Can you work these out from the drawing? Everything is in mm from the part's minimum corner. Round coordinates to 2 decimals unless told otherwise and drop trailing zeros. Loops run counter-clockwise (first coordinate to the right, second up) from the corner with the lowest first, then second, coordinate; pieces in that order, holes last. Notation, with made-up numbers: (28, 83.25) -> (51, 83.25) arc R16 ccw to (51, 92.25) -> close; hole circle Ø3 at (-18, 4.25). An arc over 180 degrees is marked (long way). One line per item, written item: value.
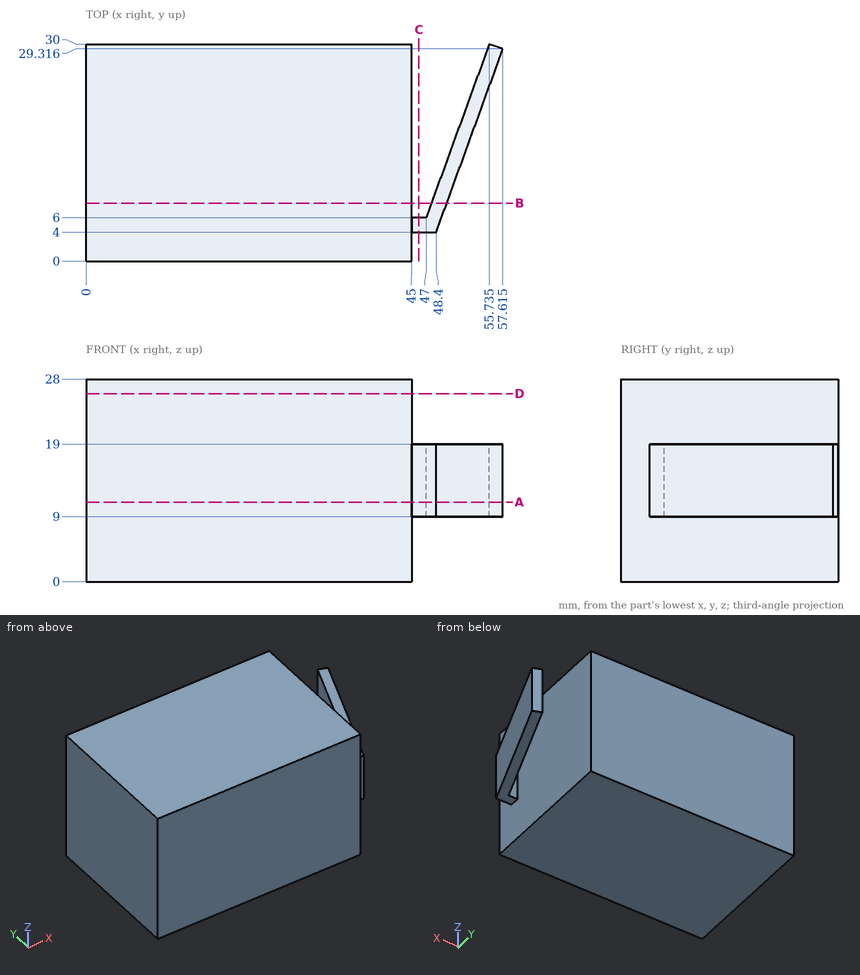
(1) If we section it at B-B, the plane y = 8: Please give me the cut outline in (x, z).
Recorded:
outline: (0, 0) -> (45, 0) -> (45, 28) -> (0, 28) -> close; (47.73, 9) -> (49.86, 9) -> (49.86, 19) -> (47.73, 19) -> close
(2) If we section it at D-D, the plane z = 26: Please give me the cut outline in (x, y), then the cut area to 3 significant figures.
Recorded:
outline: (0, 0) -> (45, 0) -> (45, 30) -> (0, 30) -> close
area: 1,350 mm²
(3) If I drill on L1, parallel to X at y = 6.5, z = 1.5; L2, parallel to X at y = 11.5, z = 12.75; L3, parallel to X at y = 21, z = 18, over which ranges is the centre line in solid material (lowest first)?
Recorded:
L1: 0 to 45
L2: 0 to 45, 49 to 51.13
L3: 0 to 45, 52.46 to 54.59
(4) If we section it at A-A, the plane z = 11: Please give me the cut outline in (x, y) (1 decimal), then the cut area to 3 significant figures.
Recorded:
outline: (0, 0) -> (45, 0) -> (45, 4) -> (48.4, 4) -> (57.6, 29.3) -> (55.7, 30) -> (47, 6) -> (45, 6) -> (45, 30) -> (0, 30) -> close
area: 1,410 mm²
(5) If we section it at C-C, the plane x = 46: Please give me the cut outline in (y, z), then the cut area to 3 significant figures.
Recorded:
outline: (4, 9) -> (6, 9) -> (6, 19) -> (4, 19) -> close
area: 20.0 mm²
(6) I'm going to push flat-ended pins straight in: pin 1 Ø4 at (x, y) = (54, 11) entering from -Z; pin 2 Ø4 at (y, z) = (23, 8.5) entering from +X; pin 3 Ø6 at (x, y) = (51.5, 22.5) entering from -Z; pin 4 Ø6.5 at (x, y) = (53, 14.5) entering from +Z. Where does each tip first touch, or does it pass through?
Recorded:
pin 1: through
pin 2: x = 56.02
pin 3: z = 9
pin 4: z = 19
